```python
from build123d import *

# Parameters (mm, degrees)
BOSS_EXTRUDE1_DEPTH = 17.78
FILLET2_R           = 5.08
SKETCH3_R           = 1.905
CUT_EXTRUDE1_DEPTH  = 43.521299369


with BuildPart() as part:
    # Sketch1 → Boss-Extrude1 (new body)
    with BuildSketch(Plane(origin=(0, 0, 0), x_dir=(0, 1, 0), z_dir=(0, 0, 1))):
        Polygon((0, 0), (0, 31.75), (6.35, 38.1), (-6.35, 38.1), (-6.35, 0), align=None)
    extrude(amount=BOSS_EXTRUDE1_DEPTH)

    # Fillet2
    # the kernel refuses this fillet: 5.08 mm, written as the material it takes off along each edge
    with BuildSketch(Plane(origin=(-38.1, -6.35, -12.7), x_dir=(0, 1, 0), z_dir=(0, 0, 1)), Plane(origin=(0, -6.35, -12.7), x_dir=(-1, 0, 0), z_dir=(0, 0, 1))) as fillet2_piece_1:
        with BuildLine():
            CenterArc((FILLET2_R, -FILLET2_R), FILLET2_R, 90, 90)
            Line((0, -FILLET2_R), (0, 0))
            Line((0, 0), (FILLET2_R, 0))
        make_face()
    extrude(amount=43.18, mode=Mode.SUBTRACT)
    with BuildSketch(Plane(origin=(0, 0, -12.7), x_dir=(-1, 0, 0), z_dir=(0, 0, 1))) as fillet2_piece_2:
        with BuildLine():
            CenterArc((FILLET2_R, FILLET2_R), FILLET2_R, 180, 90)
            Line((0, FILLET2_R), (0, 0))
            Line((0, 0), (FILLET2_R, 0))
        make_face()
    extrude(amount=43.18, mode=Mode.SUBTRACT)

    # Sketch3 → Cut-Extrude1 (cut, through all)
    with BuildSketch(Plane.XY.offset(17.78)):
        with Locations((-5.08, -3.175)):
            Circle(SKETCH3_R)
    extrude(amount=-CUT_EXTRUDE1_DEPTH, mode=Mode.SUBTRACT)


solid = part.part
```
Geometry: final body of the model. Coordinates: model frame, mm. A direction names the side the tool comes from. Round coordinates to 2 decimals unless told otherwise and drop trailing zeros. Loops run counter-clockwise (first coordinate to the right, second up) from the corner with the lowest first, then second, coordinate; pieces in that order, holes last.
Item 1: Mould query, pull axis X, two halves, no side actions, for faces 3 (the flat face through (-19, -6.35, 9)), 4 (the flat face through (-38.1, 3, 9)), 5 (the cylindrical face through (-4.201, -4.865, 9.014)), 6 (the flat face through (-34.88, 3.13, 8.77)). Classes: released by +X, released by -X, zero draft, split by the parting line, or undercut.
Checked values:
face 3: zero draft
face 4: released by -X
face 5: undercut
face 6: released by +X
Item 2: Reachability of faces 1 (the flat face through (-18, 0, 9)), 2 (the cylindrical face through (-2.28, -5.51, 8.77)) from +Z, -Z, +X, -X, +Y, -Y: full face, straight path, thin tool, end or side. Return the list, or none.
Checked values:
face 1: +Z, -Z, +X, +Y
face 2: +Z, -Z, +X, -Y
Item 3: Line query: L1, parallel to Y at x = -18, z = 16.75; L2, parallel to X at y = -3.75, z = 14.25; L3, parallel to Y at x = -3.5, z = 13. Output: solid intervals per line, ascending.
Checked values:
L1: y = -6.35 to 0
L2: x = -37.45 to -6.9, -3.26 to -0.65
L3: y = -6.1 to -4.24, -2.11 to -0.25
Item 4: Section B-B, the plane y = -4.5. Output: boundary loops of the cut face in (x, z), plus the area to 3 significant figures.
Checked values:
outline: (-36.94, 0) - (-6.45, 0) - (-6.45, 17.78) - (-36.94, 17.78) - close; (-3.71, 0) - (-1.16, 0) - (-1.16, 17.78) - (-3.71, 17.78) - close
area: 588 mm2
Item 5: Section C-C, the plane x = -15. Output: boundary loops of the cut face in (y, z), plus the area to 3 significant figures.
Checked values:
outline: (-6.35, 0) - (0, 0) - (0, 17.78) - (-6.35, 17.78) - close
area: 113 mm2
Item 6: Contact query for a flat-ended pin moving along its axis: P1, Ø9, axis at x = -21.5, z = 9, coming from the +Y side. Output: stop coordinate, or through.
Checked values:
P1: stops at y = 0
Item 7: Section A-A, the plane z = 12. Output: boundary loops of the cut face in (x, y) (3 decimals).
Checked values:
outline: (-38.1, -1.27) arc R5.08 ccw to (-33.02, -6.35) - (-5.08, -6.35) arc R5.08 ccw to (-0.371, -3.175) arc R5.08 ccw to (-5.08, 0) - (-31.75, 0) - (-38.1, 6.35) - close; hole circle Ø3.81 at (-5.08, -3.175)
